Check sheet for the modelled part. Datum: model origin and axes. Units: mm. A direction names the side the tool comes from. Give positions to 0.01 mm unless a question says otherwise; leave off trailing zeros. Loops run counter-clockwise (first coordinate to the right, second up) from the corner with the lowest first, then second, coordinate; pieces in that order, holes last. Notation, with made-up numbers: (66, 85) -> (75, 85) arc R25 ccw to (75, 100) -> close; hole circle Ø4 at (83.25, -0.5). An arc over 180 degrees is marked (long way). Write each question's results on one line, items separated by ' | '. Start each with the question number.
1. Cross-section at C-C on z = 0. Record the boundary of the cut face in (x, y), and give its area (3 significant figures).
2. Material ranges on L1, parallel to X at y = -0.25, z = 2.75; L2, parallel to X at y = 4.75, z = 0; L3, parallel to Z at x = 0, y = 4.5, recorded low to high. Write a range as from..to.
3. Tool access check on faces 5 (the face through (-1.71, 3.2, -0.38)), 6 (the face through (-4.5, -3, 0)). Record the directions out of +Z, -Z, +X, -X, +Y, -Y that give a thin tool (end or side, any length) a straight path to the whole face; none if there is none.
4. Mould release check, pull along X, two halves, no side actions. Record for faces 1 (the face through (-2, 0, 0)), 2 (the face through (10, 0, 0)), 3 (the face through (0, 6.5, 2)), 4 (the face through (-10, 0, 0)): +X half, -X half, draft (parallel to the pull), parting line (faces both ways), or undercut.
5. Gauge pin test, flat end, axial feed: pin 1 Ø4.5 at (x, z) = (-1.5, -2) entering from -Y. Record the tip position at first contact, or that the pin passes through.
6. Cross-section at B-B on y = -3.75. Record the boundary of the cut face in (x, z).
7. Cross-section at A-A on x = 0. Record the boundary of the cut face in (y, z), and give its area (4 significant figures).
8. Cross-section at D-D on y = 4.25. Record the boundary of the cut face in (x, z).
from build123d import *

# Parameters (mm, degrees)
EXTRUDE_1_DEPTH          = 5
CUT_EXTRUDE_1_DEPTH      = 18.146428199
CUT_EXTRUDE_1_DEPTH_BACK = 18.146428199
SKETCH_2_R               = 1.75


with BuildPart() as part:
    # 草图1 → 凸台-拉伸1 (new, symmetric)
    with BuildSketch(Plane.XY):
        Polygon((10, 6.5), (-10, 6.5), (-10, -6.5), (-4.5, -6.5), (-4.5, 0), (4.5, 0), (4.5, -6.5), (10, -6.5), align=None)
    extrude(amount=EXTRUDE_1_DEPTH, both=True)

    # 草图2 → 切除-拉伸1 (cut, two sides: drawn at the far end of the back side and taken through both)
    with BuildSketch(Plane(origin=(0, 6.5, 0), x_dir=(1, 0, 0), z_dir=(0, 1, 0)).offset(-CUT_EXTRUDE_1_DEPTH_BACK)):
        with Locations(Location((0, 0, 0), (0, 0, 270))):
            Circle(SKETCH_2_R)
    extrude(amount=CUT_EXTRUDE_1_DEPTH + CUT_EXTRUDE_1_DEPTH_BACK, mode=Mode.SUBTRACT)


solid = part.part
Geometry says:
1) outline: (-10, -6.5) -> (-4.5, -6.5) -> (-4.5, 0) -> (-1.75, 0) -> (-1.75, 6.5) -> (-10, 6.5) -> close; (1.75, 0) -> (4.5, 0) -> (4.5, -6.5) -> (10, -6.5) -> (10, 6.5) -> (1.75, 6.5) -> close | area: 179 mm^2
2) L1: -10..-4.5, 4.5..10 | L2: -10..-1.75, 1.75..10 | L3: -5..-1.75, 1.75..5
3) face 5: +Y, -Y | face 6: +Z, -Z, -Y
4) face 1: undercut | face 2: +X half | face 3: draft | face 4: -X half
5) pin 1: y = 0
6) outline: (-10, -5) -> (-4.5, -5) -> (-4.5, 5) -> (-10, 5) -> close; (4.5, -5) -> (10, -5) -> (10, 5) -> (4.5, 5) -> close
7) outline: (0, -5) -> (6.5, -5) -> (6.5, -1.75) -> (0, -1.75) -> close; (0, 1.75) -> (6.5, 1.75) -> (6.5, 5) -> (0, 5) -> close | area: 42.25 mm^2
8) outline: (-10, -5) -> (10, -5) -> (10, 5) -> (-10, 5) -> close; hole circle Ø3.5 at (0, 0)
